Verification items for the finished model (mm, model axes). A direction names the side the tool comes from. Give positions to 0.01 mm unless a question says otherwise; leave off trailing zeros. Write each loop counter-clockwise with the first axis right and the second up, starting at its lowest first coordinate (ties: lowest second). Pieces come first, ordered by that corner, then holes.
from build123d import *

# Parameters (mm, degrees)
F0_R     = 37.0686538278
F1_DEPTH = 102.616
F2_R     = 16.1254555479
F3_DEPTH = 147.828
F5_DEPTH = 12.7
F7_DEPTH = 17.526
F8_R     = 12.9146046276
F9_DEPTH = 296.926


with BuildPart() as f1:
    # F0 (on Top) → F1 (new body)
    with BuildSketch(Plane.XY):
        with Locations((-39.4473746419, -5.9636109509)):
            Circle(F0_R)
    extrude(amount=F1_DEPTH)

    # F2 (on face) → F3 (cut)
    with BuildSketch(Plane.XY.offset(102.616)):
        with Locations((-39.4473746419, -5.9636109509)):
            Circle(F2_R)
    extrude(amount=-F3_DEPTH, mode=Mode.SUBTRACT)

    # F4 (on face) → F5 (join)
    with BuildSketch(Plane.XY.offset(102.616)):
        with BuildLine():
            Line((72.5051784355, 31.0990400833), (-38.7802952426, 31.0990400833))
            ThreePointArc((-38.7802952426, 31.0990400833), (-13.0010815941, 20.0109666326), (-2.3787208141, -5.9636109509))
            ThreePointArc((-2.3787208141, -5.9636109509), (-13.0010815941, -31.9381885343), (-38.7802952426, -43.026261985))
            Line((-38.7802952426, -43.026261985), (75.5315870047, -43.026261985))
            ThreePointArc((75.5315870047, -43.026261985), (101.6520252983, -4.8353768612), (72.5051784355, 31.0990400833))
        make_face()
    extrude(amount=-F5_DEPTH)

    # F6 (on face) → F7 (join)
    with BuildSketch(Plane(origin=(0, 0, 0), x_dir=(1, 0, 0), z_dir=(0, 0, -1))):
        with BuildLine():
            Line((77.2129268269, 42.6493844966), (-34.133325719, 42.6493844966))
            ThreePointArc((-34.133325719, 42.6493844966), (-11.4199796813, 30.2236651208), (-2.3787208141, 5.9636109509))
            ThreePointArc((-2.3787208141, 5.9636109509), (-12.4294067676, -19.4158001643), (-37.1312376734, -31.0326132639))
            Line((-37.1312376734, -31.0326132639), (73.1777138929, -31.0326132639))
            ThreePointArc((73.1777138929, -31.0326132639), (101.6060825642, 4.3619936552), (77.2129268269, 42.6493844966))
        make_face()
    extrude(amount=-F7_DEPTH)

    # F8 (on face) → F9 (cut)
    with BuildSketch(Plane(origin=(0, 0, 0), x_dir=(1, 0, 0), z_dir=(0, 0, -1))):
        with Locations((75.1953125, 11.8927843869)):
            Circle(F8_R)
    extrude(amount=-F9_DEPTH, mode=Mode.SUBTRACT)


solid = f1.part
Item 1: Sectioned sample at C-C on x = 70. Record the cut outline in (y, z), then the cut area to 3 significant figures.
Answer key:
outline: (-43.03, 89.92) - (-23.72, 89.92) - (-23.72, 102.62) - (-43.03, 102.62) - close; (-42.65, 0) - (-23.72, 0) - (-23.72, 17.53) - (-42.65, 17.53) - close; (-0.07, 0) - (31.03, 0) - (31.03, 17.53) - (-0.07, 17.53) - close; (-0.07, 89.92) - (31.1, 89.92) - (31.1, 102.62) - (-0.07, 102.62) - close
area: 1,520 mm2
Item 2: Sectioned sample at A-A on x = 52. Record the cut outline in (y, z), then the cut area to 3 significant figures.
Answer key:
outline: (-43.03, 89.92) - (31.1, 89.92) - (31.1, 102.62) - (-43.03, 102.62) - close; (-42.65, 0) - (31.03, 0) - (31.03, 17.53) - (-42.65, 17.53) - close
area: 2,230 mm2
Item 3: Sectioned sample at B-B on y = -10. Record the cut outline in (x, z).
Answer key:
outline: (-76.3, 0) - (-55.06, 0) - (-55.06, 102.62) - (-76.3, 102.62) - close; (-23.84, 0) - (62.42, 0) - (62.42, 17.53) - (-2.6, 17.53) - (-2.6, 89.92) - (62.42, 89.92) - (62.42, 102.62) - (-23.84, 102.62) - close; (87.97, 0) - (101.51, 0) - (101.51, 17.53) - (87.97, 17.53) - close; (87.97, 89.92) - (101.52, 89.92) - (101.52, 102.62) - (87.97, 102.62) - close
Item 4: Release check for a two-part mould opening along Y. For faces 4 (the face through (101.563, -3.685, 8.64)), 5 (the face through (62.293, -12.461, 96.177)), 6 (the face through (11, -6, 0)) record: released by +Y, released by -Y, zero draft, split by the parting line, or undercut.
Answer key:
face 4: split by the parting line
face 5: undercut
face 6: zero draft
Item 5: Sectioned sample at D-D on z = 14.5. Record the cut outline in (x, y).
Answer key:
outline: (-37.13, 31.03) arc R37.07 ccw (long way) to (-34.13, -42.65) - (77.21, -42.65) arc R38.96 ccw to (73.18, 31.03) - close; hole circle Ø32.25 at (-39.45, -5.96); hole circle Ø25.83 at (75.2, -11.89)
Item 6: Set-up check for faces 1 (the face through (101.674, -5.529, 96.355)), 2 (the face through (22, -42.649, 9)), 3 (the face through (-76.48, -4.33, 50.59)): record each of +Z, -Z, +X, -X, +Y, -Y from which the full face is reachable in a straight line by a thin tool's end or side.
Answer key:
face 1: +Z, +X
face 2: -Z, +X, -Y
face 3: none
Item 7: Depth check by flat-ended pin: pin 1 (10 mm diameter, centred on x = 9.5, z = 94.5, fed in from +Y); pin 2 (5 mm diameter, centred on y = 20.5, z = 68, fed in from -X); pin 3 (2 mm diameter, centred on y = 20, z = 52, fed in from -X). Enter the tip coordinate at first touch or a pass-through.
Answer key:
pin 1: stops at y = 31.1
pin 2: stops at x = -67.73
pin 3: stops at x = -66.85
Item 8: Scan lines: line 1 along Z through (x, y) = (0, -0.5); line 2 along X through (y, z) = (-7.5, 91.5); line 3 along X through (y, z) = (7.5, 84). Record each from-to range of solid material in increasing order.
Answer key:
line 1: z = 0 to 17.53, 89.92 to 102.62
line 2: x = -76.48 to -55.5, -23.4 to 63.05, 87.34 to 101.67
line 3: x = -73.98 to -48.32, -30.57 to -4.91
